Read the model definition and answer for the solid it produces. Units are mm, in the model's axes. Round coordinates to 2 decimals unless told otherwise and drop trailing zeros. Order: outer loops, then holes, each group sorted by start corner. A loop starts at its lowest first (then second) coordinate and runs counter-clockwise, first axis right, second up. Notation, with made-up numbers: (-11, 80.25) -> (27, 80.25) arc R35 ccw to (27, 119.25) -> close; hole circle Ø10 at (30, 89). An arc over 180 degrees is marked (long way). One line per item, written item: value. Start each with the question number.
1. Consider line 1 (X direction, y = 1.45, z = -25); line 2 (X direction, y = 0.8, z = 44); line 3 (X direction, y = 2.8, z = -26). Determine where each line is inside the solid, lowest interval first.
2. Section B-B (x = -79) is taken. Give the vertices of the cut face in (y, z), then the cut area to 3 significant figures.
3. Section A-A (z = 44) is taken. Give the vertices of the cut face in (x, y).
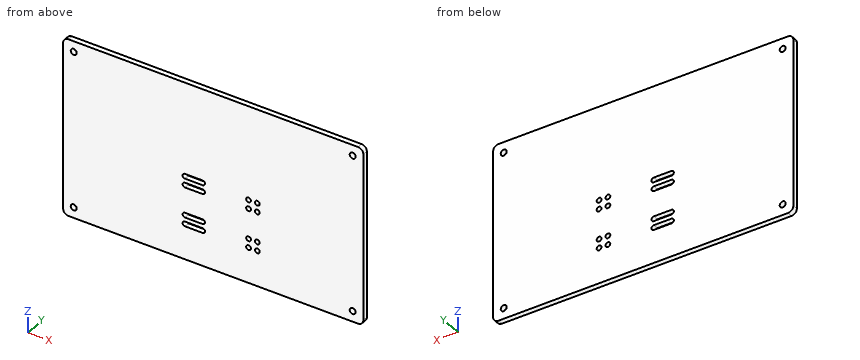
from build123d import *

# Parameters (mm, degrees)
SKETCH_1_W          = 170
SKETCH_1_H          = 100
SKETCH_1_R          = 1.7
EXTRUDE_1_DEPTH     = 3
CUT_EXTRUDE_1_REACH = 100.661
SKETCH_2_R          = 1.35
FILLET_1_R          = 3


with BuildPart() as part:
    # 草图1 → 凸台-拉伸1 (new body)
    with BuildSketch(Plane(origin=(0, 0, 0), x_dir=(1, 0, 0), z_dir=(0, 1, 0))):
        Rectangle(SKETCH_1_W, SKETCH_1_H)
        with Locations(Location((-79, -44, 0), (0, 0, 90))):
            Circle(SKETCH_1_R, mode=Mode.SUBTRACT)
        with Locations(Location((79, 44, 0), (0, 0, 90))):
            Circle(SKETCH_1_R, mode=Mode.SUBTRACT)
        with Locations(Location((79, -44, 0), (0, 0, 270))):
            Circle(SKETCH_1_R, mode=Mode.SUBTRACT)
        with Locations(Location((-79, 44, 0), (0, 0, 270))):
            Circle(SKETCH_1_R, mode=Mode.SUBTRACT)
    extrude(amount=EXTRUDE_1_DEPTH)

    # 草图2 → 切除-拉伸1 (cut, up to next)
    with BuildSketch(Plane(origin=(0, 3, 0), x_dir=(1, 0, 0), z_dir=(0, 1, 0)), mode=Mode.PRIVATE) as cut_extrude_1_sk1:
        with Locations(Location((25, 30, 0), (0, 0, 270))):
            Circle(SKETCH_2_R)
    cut_extrude_1_tool1 = extrude(cut_extrude_1_sk1.sketch, amount=-CUT_EXTRUDE_1_REACH, mode=Mode.PRIVATE) & part.part
    # 草图2 → 切除-拉伸1 (cut, up to next)
    with BuildSketch(Plane(origin=(0, 3, 0), x_dir=(1, 0, 0), z_dir=(0, 1, 0)), mode=Mode.PRIVATE) as cut_extrude_1_sk2:
        with Locations(Location((20, 30, 0), (0, 0, 270))):
            Circle(SKETCH_2_R)
    cut_extrude_1_tool2 = extrude(cut_extrude_1_sk2.sketch, amount=-CUT_EXTRUDE_1_REACH, mode=Mode.PRIVATE) & part.part
    # 草图2 → 切除-拉伸1 (cut, up to next)
    with BuildSketch(Plane(origin=(0, 3, 0), x_dir=(1, 0, 0), z_dir=(0, 1, 0)), mode=Mode.PRIVATE) as cut_extrude_1_sk3:
        with Locations(Location((25, 25, 0), (0, 0, 270))):
            Circle(SKETCH_2_R)
    cut_extrude_1_tool3 = extrude(cut_extrude_1_sk3.sketch, amount=-CUT_EXTRUDE_1_REACH, mode=Mode.PRIVATE) & part.part
    # 草图2 → 切除-拉伸1 (cut, up to next)
    with BuildSketch(Plane(origin=(0, 3, 0), x_dir=(1, 0, 0), z_dir=(0, 1, 0)), mode=Mode.PRIVATE) as cut_extrude_1_sk4:
        with Locations(Location((20, 25, 0), (0, 0, 270))):
            Circle(SKETCH_2_R)
    cut_extrude_1_tool4 = extrude(cut_extrude_1_sk4.sketch, amount=-CUT_EXTRUDE_1_REACH, mode=Mode.PRIVATE) & part.part
    # 草图2 → 切除-拉伸1 (cut, up to next)
    with BuildSketch(Plane(origin=(0, 3, 0), x_dir=(1, 0, 0), z_dir=(0, 1, 0)), mode=Mode.PRIVATE) as cut_extrude_1_sk5:
        with Locations(Location((25, 8, 0), (0, 0, 270))):
            Circle(SKETCH_2_R)
    cut_extrude_1_tool5 = extrude(cut_extrude_1_sk5.sketch, amount=-CUT_EXTRUDE_1_REACH, mode=Mode.PRIVATE) & part.part
    # 草图2 → 切除-拉伸1 (cut, up to next)
    with BuildSketch(Plane(origin=(0, 3, 0), x_dir=(1, 0, 0), z_dir=(0, 1, 0)), mode=Mode.PRIVATE) as cut_extrude_1_sk6:
        with Locations(Location((20, 8, 0), (0, 0, 270))):
            Circle(SKETCH_2_R)
    cut_extrude_1_tool6 = extrude(cut_extrude_1_sk6.sketch, amount=-CUT_EXTRUDE_1_REACH, mode=Mode.PRIVATE) & part.part
    # 草图2 → 切除-拉伸1 (cut, up to next)
    with BuildSketch(Plane(origin=(0, 3, 0), x_dir=(1, 0, 0), z_dir=(0, 1, 0)), mode=Mode.PRIVATE) as cut_extrude_1_sk7:
        with Locations(Location((25, 3, 0), (0, 0, 270))):
            Circle(SKETCH_2_R)
    cut_extrude_1_tool7 = extrude(cut_extrude_1_sk7.sketch, amount=-CUT_EXTRUDE_1_REACH, mode=Mode.PRIVATE) & part.part
    # 草图2 → 切除-拉伸1 (cut, up to next)
    with BuildSketch(Plane(origin=(0, 3, 0), x_dir=(1, 0, 0), z_dir=(0, 1, 0)), mode=Mode.PRIVATE) as cut_extrude_1_sk8:
        with Locations(Location((20, 3, 0), (0, 0, 270))):
            Circle(SKETCH_2_R)
    cut_extrude_1_tool8 = extrude(cut_extrude_1_sk8.sketch, amount=-CUT_EXTRUDE_1_REACH, mode=Mode.PRIVATE) & part.part
    # 草图2 → 切除-拉伸1 (cut, up to next)
    with BuildSketch(Plane(origin=(0, 3, 0), x_dir=(1, 0, 0), z_dir=(0, 1, 0)), mode=Mode.PRIVATE) as cut_extrude_1_sk9:
        with BuildLine():
            Line((-16, 26.35), (-6, 26.35))
            ThreePointArc((-6, 26.35), (-4.65, 25), (-6, 23.65))
            Line((-6, 23.65), (-16, 23.65))
            ThreePointArc((-16, 23.65), (-17.35, 25), (-16, 26.35))
        make_face()
    cut_extrude_1_tool9 = extrude(cut_extrude_1_sk9.sketch, amount=-CUT_EXTRUDE_1_REACH, mode=Mode.PRIVATE) & part.part
    # 草图2 → 切除-拉伸1 (cut, up to next)
    with BuildSketch(Plane(origin=(0, 3, 0), x_dir=(1, 0, 0), z_dir=(0, 1, 0)), mode=Mode.PRIVATE) as cut_extrude_1_sk10:
        with BuildLine():
            Line((-16, 31.35), (-6, 31.35))
            ThreePointArc((-6, 31.35), (-4.65, 30), (-6, 28.65))
            Line((-6, 28.65), (-16, 28.65))
            ThreePointArc((-16, 28.65), (-17.35, 30), (-16, 31.35))
        make_face()
    cut_extrude_1_tool10 = extrude(cut_extrude_1_sk10.sketch, amount=-CUT_EXTRUDE_1_REACH, mode=Mode.PRIVATE) & part.part
    # 草图2 → 切除-拉伸1 (cut, up to next)
    with BuildSketch(Plane(origin=(0, 3, 0), x_dir=(1, 0, 0), z_dir=(0, 1, 0)), mode=Mode.PRIVATE) as cut_extrude_1_sk11:
        with BuildLine():
            Line((-16, 4.35), (-6, 4.35))
            ThreePointArc((-6, 4.35), (-4.65, 3), (-6, 1.65))
            Line((-6, 1.65), (-16, 1.65))
            ThreePointArc((-16, 1.65), (-17.35, 3), (-16, 4.35))
        make_face()
    cut_extrude_1_tool11 = extrude(cut_extrude_1_sk11.sketch, amount=-CUT_EXTRUDE_1_REACH, mode=Mode.PRIVATE) & part.part
    # 草图2 → 切除-拉伸1 (cut, up to next)
    with BuildSketch(Plane(origin=(0, 3, 0), x_dir=(1, 0, 0), z_dir=(0, 1, 0)), mode=Mode.PRIVATE) as cut_extrude_1_sk12:
        with BuildLine():
            Line((-16, 9.35), (-6, 9.35))
            ThreePointArc((-6, 9.35), (-4.65, 8), (-6, 6.65))
            Line((-6, 6.65), (-16, 6.65))
            ThreePointArc((-16, 6.65), (-17.35, 8), (-16, 9.35))
        make_face()
    cut_extrude_1_tool12 = extrude(cut_extrude_1_sk12.sketch, amount=-CUT_EXTRUDE_1_REACH, mode=Mode.PRIVATE) & part.part
    add(cut_extrude_1_tool1.solids().sort_by_distance((25, 3, -30))[0], mode=Mode.SUBTRACT)
    add(cut_extrude_1_tool2.solids().sort_by_distance((20, 3, -30))[0], mode=Mode.SUBTRACT)
    add(cut_extrude_1_tool3.solids().sort_by_distance((25, 3, -25))[0], mode=Mode.SUBTRACT)
    add(cut_extrude_1_tool4.solids().sort_by_distance((20, 3, -25))[0], mode=Mode.SUBTRACT)
    add(cut_extrude_1_tool5.solids().sort_by_distance((25, 3, -8))[0], mode=Mode.SUBTRACT)
    add(cut_extrude_1_tool6.solids().sort_by_distance((20, 3, -8))[0], mode=Mode.SUBTRACT)
    add(cut_extrude_1_tool7.solids().sort_by_distance((25, 3, -3))[0], mode=Mode.SUBTRACT)
    add(cut_extrude_1_tool8.solids().sort_by_distance((20, 3, -3))[0], mode=Mode.SUBTRACT)
    add(cut_extrude_1_tool9.solids().sort_by_distance((-11, 3, -25))[0], mode=Mode.SUBTRACT)
    add(cut_extrude_1_tool10.solids().sort_by_distance((-11, 3, -30))[0], mode=Mode.SUBTRACT)
    add(cut_extrude_1_tool11.solids().sort_by_distance((-11, 3, -3))[0], mode=Mode.SUBTRACT)
    add(cut_extrude_1_tool12.solids().sort_by_distance((-11, 3, -8))[0], mode=Mode.SUBTRACT)

    # 圆角1
    fillet_1_edges = [part.edges().sort_by_distance(p)[0] for p in [
        (85, 1.5, 50),
        (-85, 1.5, 50),
        (-85, 1.5, -50),
        (85, 1.5, -50),
    ]]
    fillet(fillet_1_edges, radius=FILLET_1_R)


solid = part.part
Answer:
1. line 1: -85 to -17.35, -4.65 to 18.65, 21.35 to 23.65, 26.35 to 85
1. line 2: -85 to -80.7, -77.3 to 77.3, 80.7 to 85
1. line 3: -85 to -16.91, -5.09 to 19.09, 20.91 to 24.09, 25.91 to 85
2. outline: (0, -50) -> (3, -50) -> (3, -45.7) -> (0, -45.7) -> close; (0, -42.3) -> (3, -42.3) -> (3, 42.3) -> (0, 42.3) -> close; (0, 45.7) -> (3, 45.7) -> (3, 50) -> (0, 50) -> close
2. area: 280 mm^2
3. outline: (-85, 0) -> (-80.7, 0) -> (-80.7, 3) -> (-85, 3) -> close; (-77.3, 0) -> (77.3, 0) -> (77.3, 3) -> (-77.3, 3) -> close; (80.7, 0) -> (85, 0) -> (85, 3) -> (80.7, 3) -> close
